from build123d import *

# Parameters (mm, degrees)
ESQUISSE1_W             = 6
ESQUISSE1_H             = 6
BOSS_EXTRU_3_DEPTH      = 1.6
BOSS_EXTRU_4_DEPTH      = 1
BOSS_EXTRU_4_DEPTH_BACK = 2.6
ESQUISSE3_W             = 6
ESQUISSE3_H             = 1.5
ESQUISSE6_W             = 3
ESQUISSE6_H             = 3.6
BOSS_EXTRU_7_DEPTH      = 20


with BuildPart() as part:
    # Esquisse1 → Boss.-Extru.3 (new body)
    with BuildSketch(Plane.XY):
        with Locations((3, 3)):
            Rectangle(ESQUISSE1_W, ESQUISSE1_H)
    extrude(amount=BOSS_EXTRU_3_DEPTH)

    # Esquisse3 → Boss.-Extru.4 (add, two sides: drawn at the far end of the back side and taken through both)
    with BuildSketch(Plane.XY.offset(1.6).offset(-BOSS_EXTRU_4_DEPTH_BACK)):
        with Locations((3, 6.75)):
            Rectangle(ESQUISSE3_W, ESQUISSE3_H)
        Polygon((0, 7.5), (-1.5, 7.5), (-1.5, -1.5), (0, -1.5), (0, 0), (0, 6), align=None)
        with Locations((3, -0.75)):
            Rectangle(ESQUISSE3_W, ESQUISSE3_H)
    extrude(amount=BOSS_EXTRU_4_DEPTH + BOSS_EXTRU_4_DEPTH_BACK)

    # Esquisse6 → Boss.-Extru.7 (add)
    with BuildSketch(Plane(origin=(0, 7.5, 0), x_dir=(1, 0, 0), z_dir=(0, 1, 0))):
        with Locations((0, -0.8)):
            Rectangle(ESQUISSE6_W, ESQUISSE6_H)
    extrude(amount=BOSS_EXTRU_7_DEPTH)


solid = part.part
Geometry check sheet. Reference: the model listing, model coordinates, mm. A direction names the side the tool comes from. Round coordinates to 2 decimals unless told otherwise and drop trailing zeros. Order: outer loops, then holes, each group sorted by start corner. A loop starts at its lowest first (then second) coordinate and runs counter-clockwise, first axis right, second up. Notation, with made-up numbers: M 34.25,88.25 L 80.25,88.25 A16 ccw 80.25,94.25 Z; hole C 29,-34.75 d5. An arc over 180 degrees is marked long. Answer in a Markdown table with one row per item. Add a question column.
Item 1: Material ranges on L1, parallel to Y at x = 2, z = -0.65; L2, parallel to Z at x = 5.25, y = 5.75; L3, parallel to X at y = 10, z = 0.05, recorded low to high. Write a range as [from, to].
Item 2: Draft check along Y on faces 6 (the face through (3, 3, 1.6)), 7 (the face through (0, 27.5, 1)), 8 (the face through (1, 10, -1)). Enter one of: released by +Y, released by -Y, zero draft, split by the parting line, or undercut.
Item 3: Sectioned sample at C-C, the plane z = 2.15. Enter the section's corners in (x, y), plus the area to 3 significant figures.
Item 4: Set-up check for faces 1 (the face through (3, 0, 2)), 2 (the face through (1, 10, 2.6)), 3 (the face through (2, -1.5, 1)), 4 (the face through (4, 7.5, 1)), 5 (the face through (3, 3, 0)): record each of +Z, -Z, +X, -X, +Y, -Y from which the full face is reachable in a straight line by a thin tool's end or side.
Item 5: Sectioned sample at A-A, the plane x = 0.25. Enter the section's corners in (y, z), plus the area to 3 significant figures.
Item 6: Depth check by flat-ended pin: pin 1 Ø0.8 at (y, z) = (3, -0.5) entering from +X; pin 2 Ø1.1 at (y, z) = (4, 2) entering from +X; pin 3 Ø1.1 at (x, z) = (3.5, -0.5) entering from +Y. Enter the tip coordinate at first touch or a pass-through.
Item 7: Sectioned sample at B-B, the plane y = 1.75. Enter the section's corners in (x, z), plus the area to 3 significant figures.
Item 8: Sectioned sample at D-D, the plane x = 3.5. Enter the section's corners in (y, z), plus the area to 3 significant figures.
Filled in:
| question | item | result |
|---|---|---|
| 1 | L1 | y = [-1.5, 0], [6, 7.5] |
| 1 | L2 | z = [0, 1.6] |
| 1 | L3 | x = [-1.5, 1.5] |
| 2 | face 6 | undercut |
| 2 | face 7 | released by +Y |
| 2 | face 8 | zero draft |
| 3 | outline | M -1.5,-1.5 L 6,-1.5 L 6,0 L 0,0 L 0,6 L 6,6 L 6,7.5 L 1.5,7.5 L 1.5,27.5 L -1.5,27.5 Z |
| 3 | area | 91.5 mm² |
| 4 | face 1 | +Z, +X |
| 4 | face 2 | +Z, +X, -X, +Y, -Y |
| 4 | face 3 | +Z, -Z, +X, -X, -Y |
| 4 | face 4 | +Z, -Z, +X, +Y |
| 4 | face 5 | -Z, +X |
| 5 | outline | M -1.5,-1 L 0,-1 L 0,0 L 6,0 L 6,-1 L 27.5,-1 L 27.5,2.6 L 6,2.6 L 6,1.6 L 0,1.6 L 0,2.6 L -1.5,2.6 Z |
| 5 | area | 92.4 mm² |
| 6 | pin 1 | stops at x = 0 |
| 6 | pin 2 | stops at x = 6 |
| 6 | pin 3 | stops at y = 7.5 |
| 7 | outline | M -1.5,-1 L 0,-1 L 0,0 L 6,0 L 6,1.6 L 0,1.6 L 0,2.6 L -1.5,2.6 Z |
| 7 | area | 15.0 mm² |
| 8 | outline | M -1.5,-1 L 0,-1 L 0,0 L 6,0 L 6,-1 L 7.5,-1 L 7.5,2.6 L 6,2.6 L 6,1.6 L 0,1.6 L 0,2.6 L -1.5,2.6 Z |
| 8 | area | 20.4 mm² |
